Input: dimensioned drawing with shaded views. Units: mm. Origin: part minimum x, y, z. A direction names the side the tool comes from. Give positions to 0.01 mm unless a question says otherwise; leave off trailing zeros. Order: outer loops, then holes, each group sorted by start corner. A loop starts at its lowest first (then second) coordinate and runs counter-clockwise, first axis right, second up. Notation, with made-up numbers: (33.5, 2.5) -> (65.5, 2.5) arc R30 cw to (65.5, 36.5) -> close; hole circle Ø1 at (-35.75, 2). An arc over 180 degrees is marked (long way). Use CSV: the item, a comma, the result in double quotes.
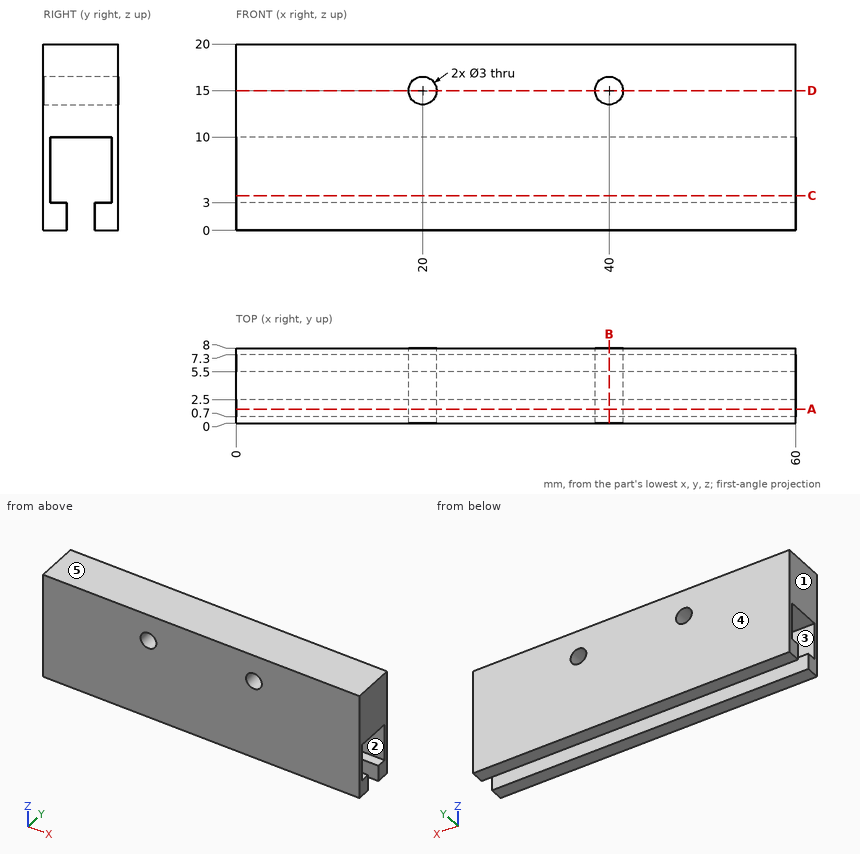
1. Section query A-A on y = 1.5. Return loops of the section in (x, z).
Answer below:
outline,"(0, 0) -> (60, 0) -> (60, 3) -> (0, 3) -> close; (0, 10) -> (60, 10) -> (60, 20) -> (0, 20) -> close; hole circle Ø3 at (20, 15); hole circle Ø3 at (40, 15)"
2. Mould query, pull axis Y, two halves, no side actions, for the marked faces 3, 4 and 5. Classes: released by +Y, released by -Y, zero draft, split by the parting line, or undercut.
Answer below:
face 3,"undercut"
face 4,"released by +Y"
face 5,"zero draft"
3. Section query C-C on z = 3.75. Return loops of the section in (x, y).
Answer below:
outline,"(0, 0) -> (60, 0) -> (60, 0.7) -> (0, 0.7) -> close; (0, 7.3) -> (60, 7.3) -> (60, 8) -> (0, 8) -> close"
4. Access query for the marked faces 1 and 2. Directions: +Z, -Z, +X, -X, +Y, -Y. A direction counts if a zero-diameter tool reaches every point of the face in a straight line with its end or side. Return the directions, or none.
Answer below:
face 1,"+Z, -Z, -X, +Y, -Y"
face 2,"+X, -X"
5. Section query B-B on x = 40. Return loops of the section in (y, z).
Answer below:
outline,"(0, 0) -> (2.5, 0) -> (2.5, 3) -> (0.7, 3) -> (0.7, 10) -> (7.3, 10) -> (7.3, 3) -> (5.5, 3) -> (5.5, 0) -> (8, 0) -> (8, 13.5) -> (0, 13.5) -> close; (0, 16.5) -> (8, 16.5) -> (8, 20) -> (0, 20) -> close"
6. Ray query, line 1 along X through (y, z) = (4.75, 15); line 2 along Y through (x, z) = (12.5, 3.25); line 3 along Y through (x, z) = (46, 2.5). Return the intervals inside material, ascending.
Answer below:
line 1,"x = 0 to 18.5, 21.5 to 38.5, 41.5 to 60"
line 2,"y = 0 to 0.7, 7.3 to 8"
line 3,"y = 0 to 2.5, 5.5 to 8"
7. Pin query (flat end, axial travel): P1, Ø5.5, axis at x = 26, z = 7.5, coming from the -Y side. Return the tip coordinate at first contact, or that it passes through.
Answer below:
P1,"stops at y = 0"
8. Section query D-D on z = 15. Return loops of the section in (x, y).
Answer below:
outline,"(0, 0) -> (18.5, 0) -> (18.5, 8) -> (0, 8) -> close; (21.5, 0) -> (38.5, 0) -> (38.5, 8) -> (21.5, 8) -> close; (41.5, 0) -> (60, 0) -> (60, 8) -> (41.5, 8) -> close"
